Verification items for the finished model (mm, model axes). A direction names the side the tool comes from. Give positions to 0.01 mm unless a question says otherwise; leave off trailing zeros. Loops run counter-clockwise (first coordinate to the right, second up) from the corner with the lowest first, then second, coordinate; pieces in that order, holes last. Notation, with made-up numbers: (16.5, 49.25) - (42.5, 49.25) arc R10 cw to (42.5, 60.25) - close; hole circle Ø1 at (18, 40.25). An arc over 180 degrees is marked (long way). One line per item, written item: value. Start each with the question number.
1. Scan lines: L1, parallel to Z at x = -4, y = 19.5; L2, parallel to Y at x = -3.5, z = 7.5; L3, parallel to Y at x = 19, z = 9.5. Record each from-to range of solid material in increasing order. Write a range as [from, to].
2. Sectioned sample at A-A (y = 0). Count the separate pieces of the cut face and the enclosed holes in it, plus the area to 3 significant figures.
3. Mould release check, pull along X, two halves, no side actions. Record for faces 3 (the cylindrical face through (-24.56, 1.774, 5.425)), 4 (the flat face through (-1, -17, 10)), 5 (the flat face through (-50, 0, 5)): pulls with the +X half, pulls with the -X half, needs draft (parallel to the pull), parting line crosses it, or undercut.
4. Gauge pin test, flat ends, axial feed: pin 1 (5 mm diameter, centred on x = 10, y = -14, fed in from +Z); pin 2 (3 mm diameter, centred on x = 17.375, y = 0, fed in from -Z); pin 3 (0.6 mm diameter, centred on x = -16.5, z = 10.5, fed in from -Y) (3 decimals). Record the tip position at first contact, or that the pin passes through.
5. Sectioned sample at D-D (x = 26). Record the cut outline in (y, z) (3 decimals), plus the area to 3 significant figures.
6. Access from +Z, -Z, +X, -X, +Y, -Y to the whole of each face (thin tool, end or side, straight path). Record for faces 1 (the flat face through (-1, 17, 10)), 2 (the cylindrical face through (24.753, 0.115, 5.425)).
7. Sectioned sample at B-B (y = -20). Record the cut outline in (x, z).
from build123d import *

# Parameters (mm, degrees)
SKETCH_W        = 100
SKETCH_H        = 50
PAD_DEPTH       = 10
SKETCH001_R     = 2
POCKET_DEPTH    = 10.001
SKETCH002_W     = 100
SKETCH002_H     = 17.75
PAD001_DEPTH    = 0.7
SKETCH003_R     = 2.625
POCKET001_DEPTH = 10.701


with BuildPart() as part:
    # Sketch → Pad (new body)
    with BuildSketch(Plane.XY):
        Rectangle(SKETCH_W, SKETCH_H)
    extrude(amount=PAD_DEPTH)

    # Sketch001 (on Face6 of Pad) → Pocket (cut, through all)
    with BuildSketch(Plane.XY.offset(10)):
        with Locations((-30, 20)):
            Circle(SKETCH001_R)
        with Locations((-30, -20)):
            Circle(SKETCH001_R)
        with Locations((30, 20)):
            Circle(SKETCH001_R)
        with Locations((30, -20)):
            Circle(SKETCH001_R)
    extrude(amount=-POCKET_DEPTH, mode=Mode.SUBTRACT)

    # Sketch002 (on Face5 of Pocket) → Pad001 (join)
    with BuildSketch(Plane.XY.offset(10)):
        Rectangle(SKETCH002_W, SKETCH002_H)
    extrude(amount=PAD001_DEPTH)

    # Sketch003 (on Face16 of Pad001) → Pocket001 (cut, through all)
    with BuildSketch(Plane.XY.offset(10.7)):
        with Locations((-32.625, 0)):
            Circle(SKETCH003_R)
        with Locations((-22.625, 0)):
            Circle(SKETCH003_R)
        with Locations((-12.625, 0)):
            Circle(SKETCH003_R)
        with Locations((-2.625, 0)):
            Circle(SKETCH003_R)
        with Locations((7.375, 0)):
            Circle(SKETCH003_R)
        with Locations((17.375, 0)):
            Circle(SKETCH003_R)
        with Locations((27.375, 0)):
            Circle(SKETCH003_R)
    extrude(amount=-POCKET001_DEPTH, mode=Mode.SUBTRACT)


solid = part.part
Results are:
1. L1: z = [0, 10]
1. L2: y = [-25, -2.47], [2.47, 25]
1. L3: y = [-25, -2.06], [2.06, 25]
2. separate pieces: 8
2. enclosed holes: 0
2. area: 677 mm^2
3. face 3: undercut
3. face 4: needs draft
3. face 5: pulls with the -X half
4. pin 1: stops at z = 10
4. pin 2: passes through
4. pin 3: stops at y = -8.875
5. outline: (-25, 0) - (-2.236, 0) - (-2.236, 10.7) - (-8.875, 10.7) - (-8.875, 10) - (-25, 10) - close; (2.236, 0) - (25, 0) - (25, 10) - (8.875, 10) - (8.875, 10.7) - (2.236, 10.7) - close
5. area: 465 mm^2
6. face 1: +Z, +X, -X, +Y
6. face 2: +Z, -Z
7. outline: (-50, 0) - (-32, 0) - (-32, 10) - (-50, 10) - close; (-28, 0) - (28, 0) - (28, 10) - (-28, 10) - close; (32, 0) - (50, 0) - (50, 10) - (32, 10) - close
